```python
from build123d import *


with BuildPart() as part:
    # Sketch1 → Revolve1 (revolve)
    with BuildSketch(Plane(origin=(0, 0, 0), x_dir=(-1, 0, 0), z_dir=(0, 0, -1)), mode=Mode.PRIVATE) as revolve1_sk:
        with BuildLine():
            Line((1.524, 3.182551134), (1.200668646, 3.567882438))
            Line((1.200668646, 3.567882438), (1.200668646, 3.6972875))
            Line((1.200668646, 3.6972875), (1.5875, 3.6972875))
            Line((1.5875, 3.6972875), (1.5875, 3.81))
            ThreePointArc((1.5875, 3.81), (1.541003202, 3.922253202), (1.42875, 3.96875))
            Line((1.42875, 3.96875), (-1.42875, 3.96875))
            ThreePointArc((-1.42875, 3.96875), (-1.541003202, 3.922253202), (-1.5875, 3.81))
            Line((-1.5875, 3.81), (-1.5875, 3.6972875))
            Line((-1.5875, 3.6972875), (-1.200668646, 3.6972875))
            Line((-1.200668646, 3.6972875), (-1.200668646, 3.567882438))
            Line((-1.200668646, 3.567882438), (-1.524, 3.182551134))
            Line((-1.524, 3.182551134), (-1.524, 2.679239625))
            Line((-1.524, 2.679239625), (-1.121293646, 2.679239625))
            Line((-1.121293646, 2.679239625), (-1.121293646, 3.6972875))
            Line((-1.121293646, 3.6972875), (-0.532839829, 3.6972875))
            ThreePointArc((-0.532839829, 3.6972875), (0, 3.921125), (0.532839829, 3.6972875))
            Line((0.532839829, 3.6972875), (1.121293646, 3.6972875))
            Line((1.121293646, 3.6972875), (1.121293646, 2.679239625))
            Line((1.121293646, 2.679239625), (1.524, 2.679239625))
            Line((1.524, 2.679239625), (1.524, 3.182551134))
        make_face()
    revolve(revolve1_sk.sketch.rotate(Axis((1.5875, 0, 0), (-1, 0, 0)), 270), axis=Axis((1.5875, 0, 0), (-1, 0, 0)))


solid = part.part
```
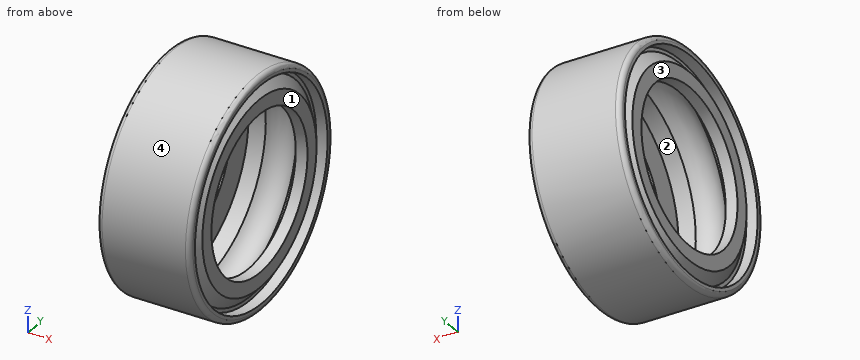
The listing builds one solid part. Answer for the finished solid, in the listing's coordinates (mm). Face numbers are marked on the shaded views. A direction names the side the tool comes from. Coordinates: 2 decimals unless noted, no trailing zeros. Write each loop counter-clockwise with the first axis right and the second up, starting at its lowest first coordinate (ties: lowest second). Pieces come first, ordered by that corner, then holes. Notation, with made-up numbers: M 51,13 L 72,13 A18 ccw 72,40 Z; hole C 88,-14 d10. An arc over 180 degrees is marked long. Use a Markdown table: item, result. Add a question column.
1. Given P1, Ø3.5, axis at y = -1.5, z = 0, coming from the +X side; P2, Ø3, axis at y = 0.5, z = 0.5, coming from the -X side; P3, Ø1, axis at x = 0, y = -2, coming from the -Z side, each flat-ended and moving along its own axis, determine where each tip first touches the part or whether it passes through.
2. For a pull along Z with two mould halves and no side action, classify the marked faces 3 and 4 as +Z half, -Z half, draft (parallel to the pull), parting line (faces both ways), or undercut.
3. Which of the six approach directions +Z, -Z, +X, -X, +Y, -Y give full straight-line access (tool end or side, diameter ignored) to the marked faces 1 and 2?
4. Section A-A (x = 0.7) is taken. Give the vertices of the cut face in (y, z), plus the area to 3 significant figures.
5. Straight lines are drawn through the part: line 1 along Y through (x, z) = (-0.95, 0); line 2 along Y through (x, z) = (-1.4, 0); line 3 along X through (y, z) = (1.5, 2.5). For each, find the intervals that lie inside material, in ascending order. Write a range as [from, to].
Data:
| question | item | result |
|---|---|---|
| 1 | P1 | stops at x = 1.52 |
| 1 | P2 | passes through |
| 1 | P3 | stops at z = -3.67 |
| 2 | face 3 | undercut |
| 2 | face 4 | parting line |
| 3 | face 1 | +X |
| 3 | face 2 | none |
| 4 | outline | C 0,0 d7.94; hole C 0,0 d7.39 |
| 4 | area | 6.54 mm2 |
| 5 | line 1 | y = [-3.97, -3.7], [3.7, 3.97] |
| 5 | line 2 | y = [-3.97, -3.7], [-3.33, -2.68], [2.68, 3.33], [3.7, 3.97] |
| 5 | line 3 | x = [-1.52, -1.12], [1.12, 1.52] |
